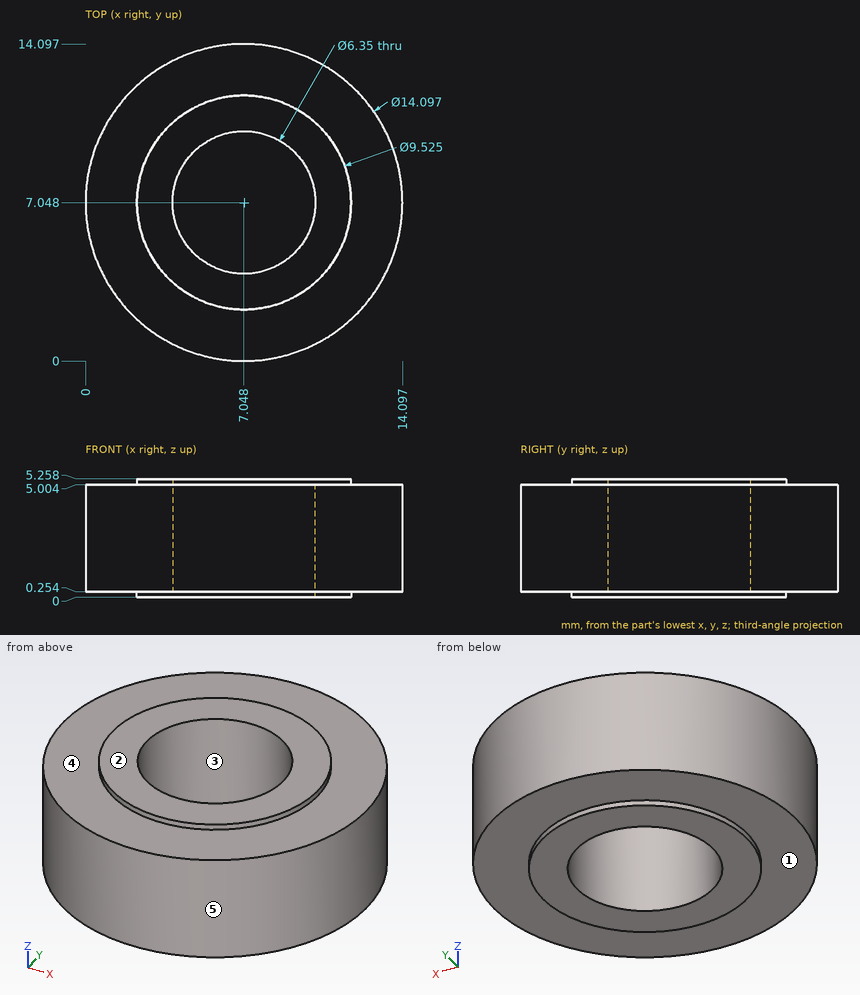
Could you check a few things on this drawing? It's one solid part, dimensions in mm from its lowest x, y, z. A direction names the side the tool comes from. Round coordinates to 2 decimals unless told otherwise and drop trailing zeros. One line per question, with ' | ' between items. Start each with the question number.
(1) Please list where these lines run through material, in increasing order: line 1 along X through (y, z) = (7, 4.55); line 2 along Z through (x, y) = (13.75, 8.75) (1 decimal); line 3 along X through (y, z) = (8.25, 1.65) (1 decimal).
(2) Thinking about a two-plate mould opening in Y: for the marked faces 3, 4 and 5, which applies, +Y half, -Y half, draft (parallel to the pull), parting line (faces both ways), or undercut?
(3) For the marked faces 1 and 2, which set-ups out of +Z, -Z, +X, -X, +Y, -Y let a thin tool reach every point of the face, with its end or its side?
(4) For P1, Ø3, axis at x = 8.5, y = 3, coming from the -Z side; P2, Ø1.5, axis at y = 3, z = 2.5, coming from the +X side; P3, Ø1.5, axis at y = 3.5, z = 2.5, coming from the -X side; P4, Ø2, axis at x = 11, z = 3.5, coming from the -Y side, each with a flat end and sliding along its axis, tell me the tip position at first contact or that it passes through.
Geometry results:
1) line 1: 0 to 3.87, 10.22 to 14.1 | line 2: 0.3 to 5 | line 3: 0.1 to 4.1, 10 to 14
2) face 3: undercut | face 4: draft | face 5: parting line
3) face 1: -Z | face 2: +Z, +X, -X, +Y, -Y
4) P1: z = 0 | P2: x = 13.28 | P3: x = 0.58 | P4: y = 0.65
